from build123d import *

# Parameters (mm, degrees)
ESQUISSE1_W        = 40
ESQUISSE1_H        = 10
MAIN_DEPTH         = 3
ESQUISSE2_W        = 40
ESQUISSE2_H        = 2.9
CENTRALFIX_DEPTH   = 1
ESQUISSE3_R        = 1.5
HOLESFIX_DEPTH     = 5
SKETCH1_W          = 3.7
SKETCH1_H          = 10
FIXSUPPORT_DEPTH   = 1.5
SKETCH2_R          = 0.8
CUT_EXTRUDE1_DEPTH = 6.5


with BuildPart() as part:
    # Esquisse1 → Main (new body)
    with BuildSketch(Plane.XY):
        with Locations((20, 5)):
            Rectangle(ESQUISSE1_W, ESQUISSE1_H)
    extrude(amount=MAIN_DEPTH)

    # Esquisse2 → CentralFix (add)
    with BuildSketch(Plane.XY.offset(3)):
        with Locations((20, 5)):
            Rectangle(ESQUISSE2_W, ESQUISSE2_H)
    extrude(amount=CENTRALFIX_DEPTH)

    # Esquisse3 → HolesFix (cut, through all)
    with BuildSketch(Plane(origin=(0, 0, 0), x_dir=(-1, 0, 0), z_dir=(0, 0, -1))):
        with Locations((-5, 5)):
            Circle(ESQUISSE3_R)
    extrude(amount=-HOLESFIX_DEPTH, mode=Mode.SUBTRACT)

    # Sketch1 → FixSupport (add)
    with BuildSketch(Plane(origin=(0, 0, 0), x_dir=(-1, 0, 0), z_dir=(0, 0, -1))):
        with Locations((-11.85, 5)):
            Rectangle(SKETCH1_W, SKETCH1_H)
        with Locations((-38.15, 5)):
            Rectangle(SKETCH1_W, SKETCH1_H)
    extrude(amount=FIXSUPPORT_DEPTH)

    # Sketch2 → Cut-Extrude1 (cut, through all)
    with BuildSketch(Plane(origin=(0, 0, -1.5), x_dir=(-1, 0, 0), z_dir=(0, 0, -1))):
        with Locations((-37.9, 5)):
            Circle(SKETCH2_R)
        with Locations((-12.1, 5)):
            Circle(SKETCH2_R)
    extrude(amount=-CUT_EXTRUDE1_DEPTH, mode=Mode.SUBTRACT)


solid = part.part
Geometry check sheet. Reference: the model listing, model coordinates, mm. A direction names the side the tool comes from. Coordinates: 2 decimals unless noted, no trailing zeros. Write each loop counter-clockwise with the first axis right and the second up, starting at its lowest first coordinate (ties: lowest second). Pieces come first, ordered by that corner, then holes. Notation, with made-up numbers: (-16, 25) -> (42, 25) arc R17 cw to (42, 52) -> close; hole circle Ø2 at (16.5, -37.75). An arc over 180 degrees is marked (long way). One line per question, with ' | ' between items.
1. Cross-section at D-D on y = 9.5. Record the cut outline in (x, z).
Answers:
outline: (0, 0) -> (10, 0) -> (10, -1.5) -> (13.7, -1.5) -> (13.7, 0) -> (36.3, 0) -> (36.3, -1.5) -> (40, -1.5) -> (40, 3) -> (0, 3) -> close
2. Depth check by flat-ended pin: pin 1 Ø0.5 at (x, z) = (1.5, 3.5) entering from -Y; pin 2 Ø6 at (x, y) = (6, 6.5) entering from -Z; pin 3 Ø0.5 at (x, z) = (21.5, 3.5) entering from +Y. Enter the tip coordinate at first touch or a pass-through.
Answers:
pin 1: stops at y = 3.55 | pin 2: stops at z = 0 | pin 3: stops at y = 6.45
3. Set-up check for faces 4 (the flat face through (2.3, 3.55, 3.5)), 5 (the flat face through (20, 8, 3)), 6 (the flat face through (10, 5, -1)), 7 (the flat face through (13.7, 5, -1)): record each of +Z, -Z, +X, -X, +Y, -Y from which the full face is reachable in a straight line by a thin tool's end or side.
Answers:
face 4: +Z, +X, -X, -Y | face 5: +Z, +X, -X, +Y | face 6: -Z, -X, +Y, -Y | face 7: -Z, +Y, -Y
4. Cross-section at C-C on x = 5. Record the cut outline in (y, z), and give its area (3 significant figures).
Answers:
outline: (0, 0) -> (3.5, 0) -> (3.5, 3) -> (0, 3) -> close; (6.5, 0) -> (10, 0) -> (10, 3) -> (6.5, 3) -> close | area: 21.0 mm²
5. Cross-section at B-B on y = 5. Record the cut outline in (x, z).
Answers:
outline: (0, 0) -> (3.5, 0) -> (3.5, 4) -> (0, 4) -> close; (6.5, 0) -> (10, 0) -> (10, -1.5) -> (11.3, -1.5) -> (11.3, 4) -> (6.5, 4) -> close; (12.9, -1.5) -> (13.7, -1.5) -> (13.7, 0) -> (36.3, 0) -> (36.3, -1.5) -> (37.1, -1.5) -> (37.1, 4) -> (12.9, 4) -> close; (38.7, -1.5) -> (40, -1.5) -> (40, 4) -> (38.7, 4) -> close
6. Cross-section at A-A on z = -0.8. Record the cut outline in (x, y).
Answers:
outline: (10, 0) -> (13.7, 0) -> (13.7, 10) -> (10, 10) -> close; (36.3, 0) -> (40, 0) -> (40, 10) -> (36.3, 10) -> close; hole circle Ø1.6 at (12.1, 5); hole circle Ø1.6 at (37.9, 5)
7. Thickness scan on probe 1 along Y at (x, z) = (12.1, 1.1); probe 2 along Y at (x, z) = (5, 1); probe 3 along Y at (x, z) = (13, 3.6). Record the ranges inside material, lowest first. Write a range as from..to.
Answers:
probe 1: y = 0..4.2, 5.8..10 | probe 2: y = 0..3.5, 6.5..10 | probe 3: y = 3.55..6.45
8. Draft check along Y on faces 1 (the flat face through (36.3, 5, -1)), 2 (the cylindrical face through (38.7, 5, 1.2)), 3 (the flat face through (20, 10, 1)). Enter one of: +Y half, -Y half, draft (parallel to the pull), parting line (faces both ways), or undercut.
Answers:
face 1: draft | face 2: undercut | face 3: +Y half
